Drawing for the job (mm, zero at the part's lowest x, y, z). Coordinates: 2 decimals unless noted, no trailing zeros. Loops run counter-clockwise (first coordinate to the right, second up) from the corner with the lowest first, then second, coordinate; pieces in that order, holes last. Notation, with made-up numbers: (15.25, 75) -> (19.25, 75) arc R30 cw to (19.25, 109) -> close; hole circle Ø10 at (69, -37). An arc over 180 degrees is marked (long way). Write each question's results on one line, items separated by ' | '.
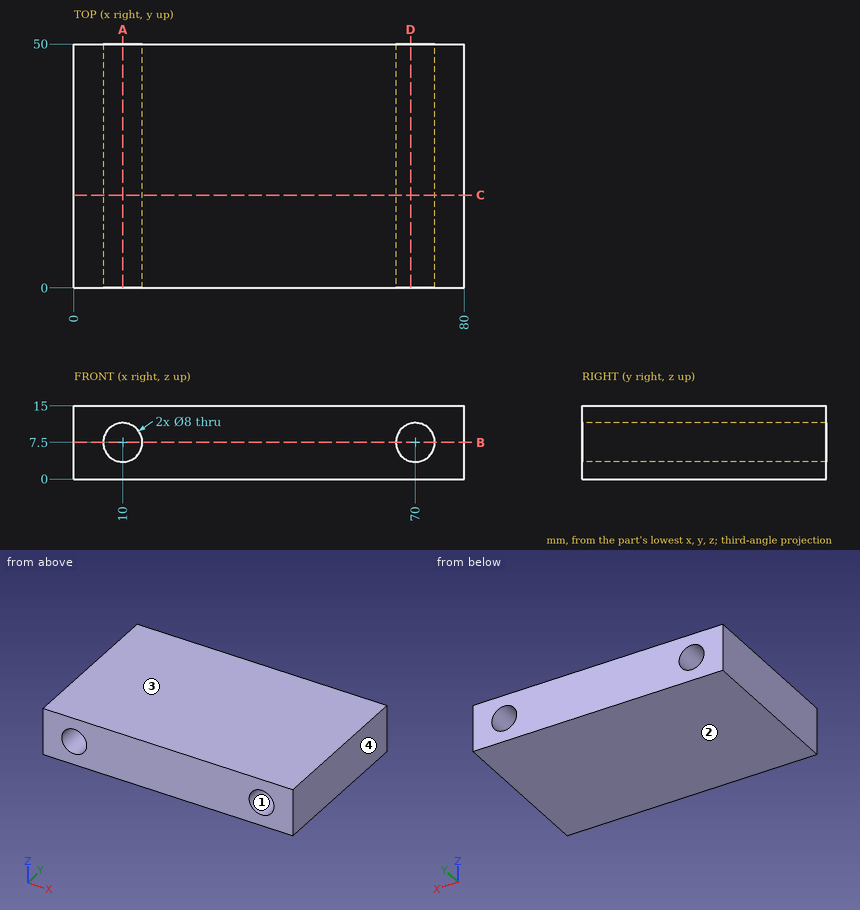
1) Slice it at C-C (y = 19). Write the cut outline in (x, z), then the cut area to 3 significant figures.
Outcome:
outline: (0, 0) -> (80, 0) -> (80, 15) -> (0, 15) -> close; hole circle Ø8 at (10, 7.5); hole circle Ø8 at (70, 7.5) | area: 1,100 mm^2
2) Pin check, flat tip, straight feed: pin 1 (4 mm diameter, centred on y = 27.5, z = 5.5, fed in from -X). Stop position of the tip, or through.
Outcome:
pin 1: stops at x = 0
3) Slice it at B-B (z = 7.5). Write the cut outline in (x, y), then the cut area to 3 significant figures.
Outcome:
outline: (0, 0) -> (6, 0) -> (6, 50) -> (0, 50) -> close; (14, 0) -> (66, 0) -> (66, 50) -> (14, 50) -> close; (74, 0) -> (80, 0) -> (80, 50) -> (74, 50) -> close | area: 3,200 mm^2
4) Two-plate mould, pull along Z, no slides. Class the marked faces 1, 2, 3 and 4: pulls with the +Z half, pulls with the -Z half, needs draft (parallel to the pull), parting line crosses it, or undercut.
Outcome:
face 1: undercut | face 2: pulls with the -Z half | face 3: pulls with the +Z half | face 4: needs draft
5) Slice it at A-A (x = 10). Write the cut outline in (y, z), then the cut area to 3 significant figures.
Outcome:
outline: (0, 0) -> (50, 0) -> (50, 3.5) -> (0, 3.5) -> close; (0, 11.5) -> (50, 11.5) -> (50, 15) -> (0, 15) -> close | area: 350 mm^2
6) Drill centre lines: L1, parallel to X at y = 5, z = 7.75; L2, parallel to Z at x = 70, y = 11; L3, parallel to X at y = 11.5, z = 10. Where is each one in solid material? Low to high. Write a range as from..to.
Outcome:
L1: x = 0..6.01, 13.99..66.01, 73.99..80 | L2: z = 0..3.5, 11.5..15 | L3: x = 0..6.88, 13.12..66.88, 73.12..80
7) Slice it at D-D (x = 69). Write the cut outline in (y, z).
Outcome:
outline: (0, 0) -> (50, 0) -> (50, 3.63) -> (0, 3.63) -> close; (0, 11.37) -> (50, 11.37) -> (50, 15) -> (0, 15) -> close
